Autodesk Inventor part; units mm, degrees
ref_plane "Work Plane1" through (29, 0, 0) normal (0, -1, 0) x (1, 0, 0)
ref_plane "YZ Plane" through (0, 0, 0) normal (1, 0, 0) x (0, 1, 0)
ref_plane "XZ Plane" through (0, 0, 0) normal (0, 1, 0) x (-1, 0, 0)
sketch "Sketch1" plane through (0, 0, 0) normal (0, 0, 1) x (1, 0, 0)
  line L0 (-1, 0) -> (35, 0)
  line L1 (35, 0) -> (35, 2)
  line L2 (35, 2) -> (15, 2)
  line L3 (15, 2) -> (14.5705, 2)
  line L4 (14.5705, 2) -> (0, 2)
  line L5 (0, 2) -> (0, 3.5)
  line L6 (0, 3.5) -> (-4, 3.5)
  line L7 (-4, 3.5) -> (-4, 1.7321)
  line L8 (-4, 1.7321) -> (-2, 1.7321)
  line L9 (-2, 1.7321) -> (-1, 0)
  line L10 (-11.8, 0) -> (42.8, 0)
  line L11 (0, -0.7) -> (0, 4.2)
  line L12 (15, 2) -> (0, 2) construction
  dimension "d1" = 20
  dimension "d2" = 0.4295
  dimension "d3" = 4
  dimension "d4" = 2
  dimension "d5" = 60
  dimension "d6" = 4
  dimension "d7" = 4
  dimension "d8" = 3.4641
  dimension "d9" = 7
  dimension "d26" = 35
revolve "Body" add sketch "Sketch1" angle 360 about axis through (-1, 0, 0) along (1, 0, 0)
sketch "Sketch2" plane through (-4, 0, 0) normal (-1, 0, 0) x (0, 0, 1)
  circle A0 centre (0, 0) radius 1.7321
  line L0 (0, -4.9) -> (0, 4.9)
  line L1 (-4.9, 0) -> (4.9, 0)
  line L2 (1.7321, 0) -> (0.866, -1.5)
  line L3 (0.866, -1.5) -> (-0.866, -1.5)
  line L4 (-0.866, -1.5) -> (-1.7321, 0)
  line L5 (-1.7321, 0) -> (-0.866, 1.5)
  line L6 (-0.866, 1.5) -> (0.866, 1.5)
  line L7 (0.866, 1.5) -> (1.7321, 0)
extrude "Slot" add sketch "Sketch2" against normal up to next contours L7 A0 | A0 L2 | L6 L0 A0 | A0 L0 L3 | L0 L6 A0 | A0 L3 L0 | L4 A0 | A0 L5
fillet "Fillet1" radius 0.4 1 edges at (-4, -3.5, 0)
thread "Thread"
chamfer "Chamfer1" distance 0.4294 distance2 0.4294 1 edges at (35, -2, 0) measured on face at (35, 0.0262, -0.4421)
ref_plane "Work Plane1" through (29, 0, 0) normal (0, -1, 0) x (1, 0, 0)
fillet "Fillet2" radius 0.1 1 edges at (0, -2, 0)
equation "\"d30\" = R"
equation "\"d17\" = RR"
equation "\"d13\" = GEL"
equation "\"d15\" = -0.5 * SPD + 0.5 * GD"
equation "\"d16\" = GUL"
equation "\"d1\" = GEL"
equation "\"d3\" = KOH"
equation "\"d4\" = INTI"
equation "\"d6\" = GD"
equation "\"d7\" = BDM"
equation "\"d8\" = 1.1547 * SW"
equation "\"d9\" = KOD"
equation "\"d26\" = NLG"
equation "\"GD\" = 4"
equation "\"NLG\" = 35"
equation "\"GEL\" = 20"
equation "\"KOD\" = 7"
equation "\"KOH\" = 4"
equation "\"INTI\" = 2"
equation "\"GAL\" = 0.61345 * PTC"
equation "\"GUL\" = 0.61345 * PTC"
equation "\"BDM\" = NND"
equation "\"SW\" = 3"
equation "\"RR\" = 0.4"
equation "\"SPD\" = NND - 1.2269 * PTC"
equation "\"R\" = 0.1"
equation "\"TOA\" = 30deg"
equation "\"GD1\" = THREADDIA - 1.2269 * PTC"
equation "\"THREADDIA\" = 4"
equation "\"FAWI\" = 45deg"
equation "\"PTC\" = 0.7"
equation "\"NND\" = 4"
equation "\"E0\" = 1.155 * SW"
properties part number "ISO 4762  - M4 x 35" material "Stainless Steel, 440C"
Here's how the part is built. I have some questions about the finished solid (model axes, mm). A direction names the side the tool comes from. Round coordinates to 2 decimals unless told otherwise and drop trailing zeros. Write each loop counter-clockwise with the first axis right and the second up, starting at its lowest first coordinate (ties: lowest second). Pieces come first, ordered by that corner, then holes.
Q1. Which directions (+Z, -Z, +X, -X, +Y, -Y) give clear straight access to the entire face, cutting with the end or side of a thin tool? Please do faces 1 (the flat face through (-2.948, 0.761, 1.293)), 2 (the cylindrical face through (17, 0, 2)), 3 (the flat face through (35, 0, 0)).
Q2. Will these pins go through, and if not, where does the flat tip stop? P1, Ø2, axis at x = 15, z = -0.5, coming from the +Y side; P2, Ø1.5, axis at x = 9.5, y = 1, coming from the +Z side; P3, Ø1.5, axis at x = 11.5, y = 0, coming from the -Z side.
Q3. If we section it at A-A on x = 28.5: Write out the boundary of the cut face in (y, z).
Q4. Please list where these lines run through material, in increasing order: probe 1 along Y at (x, z) = (13, -1); probe 2 along X at (y, z) = (-0.25, 3); probe 3 along X at (y, z) = (0.5, 0.75).
Q5. If we mould it in two halves opening along Y, with no side actions, what happens to faces 4 (the flat face through (-3, -1.5, 0)), 5 (the cylindrical face through (-1.825, 3.233, 1.341)), 6 (the conical face through (-1, 0, 0)), 7 (the flat face through (0, 2, -2))? For each: +Y half, -Y half, draft (parallel to the pull), parting line (faces both ways), or undercut.
Answer below:
1. face 1: -X
1. face 2: +X
1. face 3: +Z, -Z, +X, +Y, -Y
2. P1: stops at y = 2
2. P2: stops at z = 1.98
2. P3: stops at z = -2
3. outline: circle Ø4 at (0, 0)
4. probe 1: y = -1.73 to 1.73
4. probe 2: x = -4 to 0
4. probe 3: x = -1.52 to 35
5. face 4: undercut
5. face 5: parting line
5. face 6: undercut
5. face 7: draft
